The model under review builds one solid part; all positions refer to its coordinate system, in mm. A direction names the side the tool comes from. Give positions to 0.01 mm unless a question says otherwise; leave off trailing zeros. Loops run counter-clockwise (first coordinate to the right, second up) from the corner with the lowest first, then second, coordinate; pieces in that order, holes last. Notation, with made-up numbers: M -27.5,46 L -17.5,46 A30 cw -17.5,78 Z; hole C 85,-26 d7. An arc over 180 degrees is marked long. Put each result on its own line as item: value. Start each with the question number.
from build123d import *

# Parameters (mm, degrees)
SKETCH1_W           = 3.7
SKETCH1_H           = 5.5
BOSS_EXTRUDE1_DEPTH = 6
SKETCH3_W           = 9.478987056
SKETCH3_H           = 10.898659885
SKETCH3_W_2         = 3.7
SKETCH3_H_2         = 5.5
BOSS_EXTRUDE2_DEPTH = 8.5


with BuildPart() as part:
    # Sketch1 → Boss-Extrude1 (new body)
    with BuildSketch(Plane.XY):
        with BuildLine():
            Line((4.85, 5.75), (4.85, -5.75))
            Line((4.85, -5.75), (-4.628987056, -5.75))
            Line((-4.628987056, -5.75), (-4.628987056, 5.148659885))
            ThreePointArc((-4.628987056, 5.148659885), (11.538438682, 26.332485721), (38.123219895, 28.173556039))
            ThreePointArc((38.123219895, 28.173556039), (45.046416869, 16.141331151), (46.440789316, 2.329712217))
            Line((46.440789316, 2.329712217), (41.93897109, 2.329712217))
            ThreePointArc((41.93897109, 2.329712217), (40.981754891, 14.299726349), (35.619891873, 25.044396012))
            ThreePointArc((35.619891873, 25.044396012), (15.392209294, 23.120190877), (4.85, 5.75))
        make_face()
        Rectangle(SKETCH1_W, SKETCH1_H, mode=Mode.SUBTRACT)
    extrude(amount=BOSS_EXTRUDE1_DEPTH)

    # Sketch3 → Boss-Extrude2 (add)
    with BuildSketch(Plane.XY):
        with Locations((0.110506472, -0.300670057)):
            Rectangle(SKETCH3_W, SKETCH3_H)
        Rectangle(SKETCH3_W_2, SKETCH3_H_2, mode=Mode.SUBTRACT)
    extrude(amount=-BOSS_EXTRUDE2_DEPTH)


solid = part.part
(1) To check wall thickness, follow L1, parallel to X at y = -2, z = -7.5; L2, parallel to Z at x = 32, y = 27; L3, parallel to X at y = 3, z = -7. State the ranges of each line that lie inside material, in increasing order. Write a range as [from, to].
(2) We need section C-C, the plane z = -7. Write out the cut boundary in (x, y).
(3) For faces 1 (the flat face through (4.85, 0, -1)), 2 (the flat face through (0, 5.149, -4)), 3 (the flat face through (44, 2.33, 3)), 4 (the flat face through (-1.85, 0, -1)), list the 3-axis set-ups (+Z, -Z, +X, -X, +Y, -Y) from which the entire face can be reached by the end or side of a thin tool; tool diameter is ignored.
(4) We need section B-B, the plane z = 2.25. Write out the cut boundary in (x, y).
(5) We need section D-D, the plane y = 20. Write out the cut boundary in (x, z), plus the area to 3 significant figures.
(6) Insertion check: pin 1 (12 mm diameter, centred on x = 25.5, y = 21, fed in from -Z); pin 2 (3 mm diameter, centred on x = -1, z = -3.5, fed in from +Y); pin 3 (5 mm diameter, centred on x = 43, z = 2.5, fed in from -Y). Each pin has a flat end and moves straight along its axis. Give the tip position at first contact, or say it passes through.
(7) We need section A-A, the plane y = -1.5. Write out the cut boundary in (x, z), plus the area to 3 significant figures.
(8) Draft analysis for pull direction Y (two halves, no side actions). For faces 5 (the cylindrical face through (11.201, 26.148, 2.958)), 6 (the flat face through (17, 25, 0)), 7 (the cylindrical face through (41.027, 14.137, 2.958)), state which applies: +Y half, -Y half, draft (parallel to the pull), parting line (faces both ways), or undercut.
Check sheet entries:
1. L1: x = [-4.63, -1.85], [1.85, 4.85]
1. L2: z = [0, 6]
1. L3: x = [-4.63, 4.85]
2. outline: M -4.63,-5.75 L 4.85,-5.75 L 4.85,5.15 L -4.63,5.15 Z; hole M -1.85,-2.75 L 1.85,-2.75 L 1.85,2.75 L -1.85,2.75 Z
3. face 1: +Z, -Z, -Y
3. face 2: -Z, +X, -X, +Y
3. face 3: +Z, -Z, +X, -Y
3. face 4: +Z, -Z
4. outline: M -4.63,-5.75 L 4.85,-5.75 L 4.85,5.75 A22.65 cw 35.62,25.04 A31.54 cw 41.94,2.33 L 46.44,2.33 A33.18 ccw 38.12,28.17 A32.32 ccw -4.63,5.15 Z; hole M -1.85,-2.75 L 1.85,-2.75 L 1.85,2.75 L -1.85,2.75 Z
5. outline: M 3.3,0 L 11.46,0 L 11.46,6 L 3.3,6 Z; M 38.78,0 L 43.53,0 L 43.53,6 L 38.78,6 Z
5. area: 77.5 mm²
6. pin 1: stops at z = 0
6. pin 2: stops at y = 5.15
6. pin 3: stops at y = 2.33
7. outline: M -4.63,-8.5 L -1.85,-8.5 L -1.85,6 L -4.63,6 Z; M 1.85,-8.5 L 4.85,-8.5 L 4.85,6 L 1.85,6 Z
7. area: 83.8 mm²
8. face 5: +Y half
8. face 6: draft
8. face 7: undercut
